Read the model definition and answer for the solid it produces. Units are mm, in the model's axes. Face numbers are marked on the shaded views. A direction names the side the tool comes from. Coordinates: 2 decimals unless noted, no trailing zeros. Write each loop counter-clockwise with the first axis right and the second up, starting at its lowest first coordinate (ties: lowest second). Pieces come first, ordered by that corner, then holes. Notation, with made-up numbers: (-6.5, 83.5) - (36.5, 83.5) arc R19 ccw to (36.5, 100.5) - close; hole circle Ø1 at (1.5, -39). An arc over 180 degrees is marked (long way). Return JSON: item names as keys, results as strings.
```python
from build123d import *

# Parameters (mm, degrees)
SKETCH1_R           = 50
BOSS_EXTRUDE1_DEPTH = 10
SKETCH2_R           = 20
CUT_EXTRUDE1_DEPTH  = 5
CUT_EXTRUDE6_DEPTH  = 3
SKETCH8_R           = 1.7
CUT_EXTRUDE7_DEPTH  = 10
BOSS_EXTRUDE3_DEPTH = 10
CUT_EXTRUDE11_DEPTH = 10
SKETCH15_W          = 131.735170003
SKETCH15_H          = 179.266555965
CUT_EXTRUDE12_DEPTH = 79
BOSS_EXTRUDE4_DEPTH = 4.9
SKETCH17_R          = 1.7
CUT_EXTRUDE13_DEPTH = 10
CUT_EXTRUDE14_DEPTH = 3
SKETCH19_W          = 78.571428572
SKETCH19_H          = 5.1
CUT_EXTRUDE15_DEPTH = 0.5
CUT_EXTRUDE16_DEPTH = 10
CUT_EXTRUDE17_DEPTH = 5.1
SKETCH24_R          = 1.7
CUT_EXTRUDE19_DEPTH = 5.1
SKETCH25_R          = 11
CUT_EXTRUDE20_DEPTH = 7.2
SKETCH26_R          = 9
CUT_EXTRUDE21_DEPTH = 7.2
SKETCH27_R          = 3
CUT_EXTRUDE22_DEPTH = 11
SKETCH28_R          = 1.6
CUT_EXTRUDE23_DEPTH = 12
SKETCH29_R          = 2.9
SKETCH29_R_2        = 1.6
CUT_EXTRUDE24_DEPTH = 3.5
SKETCH30_R          = 12
CUT_EXTRUDE25_DEPTH = 2.4
SKETCH31_R          = 2.8
CUT_EXTRUDE26_DEPTH = 3
FILLET1_R           = 20


with BuildPart() as part:
    # Sketch1 → Boss-Extrude1 (new body)
    with BuildSketch(Plane(origin=(0, 0, 0), x_dir=(1, 0, 0), z_dir=(0, 1, 0))):
        Circle(SKETCH1_R)
    extrude(amount=BOSS_EXTRUDE1_DEPTH)

    # Sketch2 → Cut-Extrude1 (cut)
    with BuildSketch(Plane(origin=(0, 10, 0), x_dir=(1, 0, 0), z_dir=(0, 1, 0))):
        Circle(SKETCH2_R)
    extrude(amount=-CUT_EXTRUDE1_DEPTH, mode=Mode.SUBTRACT)

    # Sketch7 → Cut-Extrude6 (cut)
    with BuildSketch(Plane.XZ):
        with BuildLine():
            ThreePointArc((-2.85, 14.726761355), (0, 15), (2.85, 14.726761355))
            Line((2.85, 14.726761355), (2.85, 16.645448267))
            Line((2.85, 16.645448267), (0, 18.290896534))
            Line((0, 18.290896534), (-2.85, 16.645448267))
            Line((-2.85, 16.645448267), (-2.85, 14.726761355))
        make_face()
        with BuildLine():
            Line((2.85, 13.354551733), (2.85, 14.726761355))
            ThreePointArc((2.85, 14.726761355), (0, 15), (-2.85, 14.726761355))
            Line((-2.85, 14.726761355), (-2.85, 13.354551733))
            Line((-2.85, 13.354551733), (0, 11.709103466))
            Line((0, 11.709103466), (2.85, 13.354551733))
        make_face()
        Polygon((-12.990381057, -4.209103466), (-15.840381057, -5.854551733), (-15.840381057, -9.145448267), (-12.990381057, -10.790896534), (-10.140381057, -9.145448267), (-10.140381057, -5.854551733), align=None)
        Polygon((15.840381057, -5.854551733), (12.990381057, -4.209103466), (10.140381057, -5.854551733), (10.140381057, -9.145448267), (12.990381057, -10.790896534), (15.840381057, -9.145448267), align=None)
    extrude(amount=-CUT_EXTRUDE6_DEPTH, mode=Mode.SUBTRACT)

    # Sketch8 → Cut-Extrude7 (cut)
    with BuildSketch(Plane.XZ):
        with Locations((0, 15)):
            Circle(SKETCH8_R)
        with Locations((12.990381057, -7.5)):
            Circle(SKETCH8_R)
        with Locations((-12.990381057, -7.5)):
            Circle(SKETCH8_R)
    extrude(amount=-CUT_EXTRUDE7_DEPTH, mode=Mode.SUBTRACT)


with BuildPart() as body_2:
    # Sketch9 → Boss-Extrude3 (new body)
    with BuildSketch(Plane.XZ):
        with BuildLine():
            Line((-50, 350), (-50, 0))
            ThreePointArc((-50, 0), (0, 50), (50, 0))
            Line((50, 0), (50, 350))
            Line((50, 350), (-50, 350))
        make_face()
    extrude(amount=-BOSS_EXTRUDE3_DEPTH)

    # Sketch13 → Cut-Extrude11 (cut)
    with BuildSketch(Plane.XZ):
        with BuildLine():
            Line((-50, 350), (-50, 0))
            ThreePointArc((-50, 0), (-49.817332452, 4.270057067), (-49.270664506, 8.5089141))
            Line((-49.270664506, 8.5089141), (-20, 350))
            Line((-20, 350), (-50, 350))
        make_face()
        with BuildLine():
            Line((20, 350), (49.270664506, 8.5089141))
            ThreePointArc((49.270664506, 8.5089141), (49.817332452, 4.270057067), (50, 0))
            Line((50, 0), (50, 350))
            Line((50, 350), (20, 350))
        make_face()
    extrude(amount=-CUT_EXTRUDE11_DEPTH, mode=Mode.SUBTRACT)


with BuildPart() as cut_extrude12_tool:
    # Sketch15 → Cut-Extrude12 (new body)
    with BuildSketch(Plane(origin=(0, 10, 0), x_dir=(1, 0, 0), z_dir=(0, 1, 0))):
        with Locations((-8.166136658, -35.366722018)):
            Rectangle(SKETCH15_W, SKETCH15_H)
    extrude(amount=-CUT_EXTRUDE12_DEPTH)


with BuildPart() as part_1:
    add(part.part)

    # Cut-Extrude12: cut by cut_extrude12_tool
    add(cut_extrude12_tool.part, mode=Mode.SUBTRACT)


with BuildPart() as body_2_1:
    add(body_2.part)

    # Cut-Extrude12: cut by cut_extrude12_tool
    add(cut_extrude12_tool.part, mode=Mode.SUBTRACT)

    # Sketch16 → Boss-Extrude4 (add)
    with BuildSketch(Plane(origin=(0, 10, 0), x_dir=(1, 0, 0), z_dir=(0, 1, 0))):
        Polygon((40.972386827, -105.322153681), (-40.972386827, -105.322153681), (-39.285714286, -125), (39.285714286, -125), align=None)
    extrude(amount=-BOSS_EXTRUDE4_DEPTH)

    # Sketch17 → Cut-Extrude13 (cut)
    with BuildSketch(Plane.XZ.offset(-5.1)):
        with Locations((-25, 115)):
            Circle(SKETCH17_R)
        with Locations((25, 115)):
            Circle(SKETCH17_R)
    extrude(amount=-CUT_EXTRUDE13_DEPTH, mode=Mode.SUBTRACT)

    # Sketch18 → Cut-Extrude14 (cut)
    with BuildSketch(Plane(origin=(0, 10, 0), x_dir=(1, 0, 0), z_dir=(0, 1, 0))):
        Polygon((-25, -111.651368439), (-27.9, -113.325684219), (-27.9, -116.674315781), (-25, -118.348631561), (-22.1, -116.674315781), (-22.1, -113.325684219), align=None)
        Polygon((22.1, -113.325684219), (25, -111.651368439), (27.9, -113.325684219), (27.9, -116.674315781), (25, -118.348631561), (22.1, -116.674315781), align=None)
    extrude(amount=-CUT_EXTRUDE14_DEPTH, mode=Mode.SUBTRACT)

    # Sketch19 → Cut-Extrude15 (cut)
    with BuildSketch(Plane(origin=(0, 0, 125), x_dir=(-1, 0, 0), z_dir=(0, 0, -1))):
        with Locations((0, 2.55)):
            Rectangle(SKETCH19_W, SKETCH19_H)
    extrude(amount=-CUT_EXTRUDE15_DEPTH, mode=Mode.SUBTRACT)

    # Sketch21 → Cut-Extrude16 (cut)
    with BuildSketch(Plane.XZ):
        Polygon((30.285714286, 230), (-30.285714286, 230), (-39.242857143, 125.5), (39.242857143, 125.5), align=None)
        Polygon((-30.285714286, 230), (-45.620097138, 230), (-45.620097138, 89.112609713), (46.495880164, 89.112609713), (46.495880164, 230), (30.285714286, 230), (39.242857143, 125.5), (-39.242857143, 125.5), align=None)
    extrude(amount=-CUT_EXTRUDE16_DEPTH, mode=Mode.SUBTRACT)

    # Sketch21_3 → Cut-Extrude17 (cut)
    with BuildSketch(Plane.XZ):
        Polygon((-28.571428571, 250), (-30.285714286, 230), (30.285714286, 230), (28.571428571, 250), align=None)
    extrude(amount=-CUT_EXTRUDE17_DEPTH, mode=Mode.SUBTRACT)

    # Sketch24 → Cut-Extrude19 (cut)
    with BuildSketch(Plane.XZ.offset(-5.1)):
        with Locations((20, 240)):
            Circle(SKETCH24_R)
        with Locations((-20, 240)):
            Circle(SKETCH24_R)
    extrude(amount=-CUT_EXTRUDE19_DEPTH, mode=Mode.SUBTRACT)

    # Sketch25 → Cut-Extrude20 (cut)
    with BuildSketch(Plane.XZ):
        with Locations((0, 330)):
            Circle(SKETCH25_R)
    extrude(amount=-CUT_EXTRUDE20_DEPTH, mode=Mode.SUBTRACT)

    # Sketch26 → Cut-Extrude21 (cut)
    with BuildSketch(Plane.XZ.offset(-7.2)):
        with Locations((0, 330)):
            Circle(SKETCH26_R)
    extrude(amount=-CUT_EXTRUDE21_DEPTH, mode=Mode.SUBTRACT)

    # Sketch27 → Cut-Extrude22 (cut)
    with BuildSketch(Plane.XZ):
        with Locations((0, 270)):
            Circle(SKETCH27_R)
    extrude(amount=-CUT_EXTRUDE22_DEPTH, mode=Mode.SUBTRACT)

    # Sketch28 → Cut-Extrude23 (cut)
    with BuildSketch(Plane(origin=(0, 10, 0), x_dir=(1, 0, 0), z_dir=(0, 1, 0))):
        with Locations((-15.5, -254.5)):
            Circle(SKETCH28_R)
        with Locations((15.5, -254.5)):
            Circle(SKETCH28_R)
        with Locations((15.5, -285.5)):
            Circle(SKETCH28_R)
        with Locations((-15.5, -285.5)):
            Circle(SKETCH28_R)
    extrude(amount=-CUT_EXTRUDE23_DEPTH, mode=Mode.SUBTRACT)

    # Sketch29 → Cut-Extrude24 (cut)
    with BuildSketch(Plane.XZ):
        with Locations((-15.5, 285.5)):
            Circle(SKETCH29_R)
        with Locations((-15.5, 285.5)):
            Circle(SKETCH29_R_2, mode=Mode.SUBTRACT)
        with Locations((15.5, 285.5)):
            Circle(SKETCH29_R)
        with Locations((15.5, 254.5)):
            Circle(SKETCH29_R)
        with Locations((-15.5, 254.5)):
            Circle(SKETCH29_R)
    extrude(amount=-CUT_EXTRUDE24_DEPTH, mode=Mode.SUBTRACT)

    # Sketch30 → Cut-Extrude25 (cut)
    with BuildSketch(Plane(origin=(0, 10, 0), x_dir=(1, 0, 0), z_dir=(0, 1, 0))):
        with Locations((0, -270)):
            Circle(SKETCH30_R)
    extrude(amount=-CUT_EXTRUDE25_DEPTH, mode=Mode.SUBTRACT)

    # Sketch31 → Cut-Extrude26 (cut)
    with BuildSketch(Plane(origin=(0, 10, 0), x_dir=(1, 0, 0), z_dir=(0, 1, 0))):
        with Locations((-20, -240)):
            Circle(SKETCH31_R)
        with Locations((20, -240)):
            Circle(SKETCH31_R)
    extrude(amount=-CUT_EXTRUDE26_DEPTH, mode=Mode.SUBTRACT)

    # Fillet1
    fillet1_edges = [body_2_1.edges().sort_by_distance(p)[0] for p in [
        (-20, 5, 350),
        (20, 5, 350),
    ]]
    fillet(fillet1_edges, radius=FILLET1_R)


solid = body_2_1.part
```
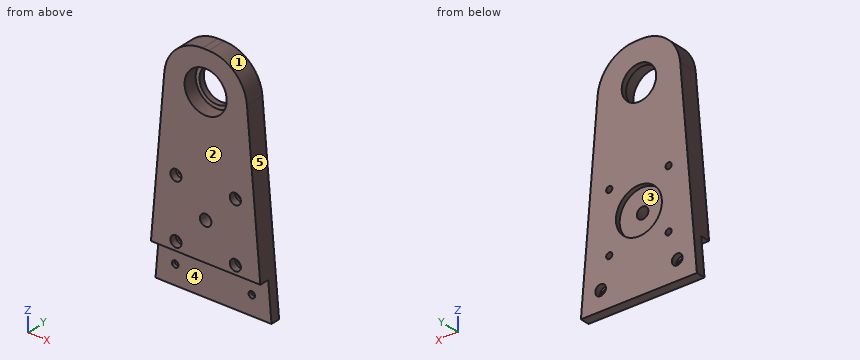
(1) A cutting plane is placed at C-C (z = 270). Determine the outline of the cut face in (x, y).
Answer:
{"outline": "(-26.86, 0) - (-3, 0) - (-3, 7.6) - (-12, 7.6) - (-12, 10) - (-26.86, 10) - close; (3, 0) - (26.86, 0) - (26.86, 10) - (12, 10) - (12, 7.6) - (3, 7.6) - close"}
(2) A cutting plane is placed at D-D (x = 15.5). Determine the outline of the cut face in (y, z).
Answer:
{"outline": "(0, 250) - (5.1, 250) - (5.1, 230) - (10, 230) - (10, 252.9) - (3.5, 252.9) - (3.5, 251.6) - (0, 251.6) - close; (0, 257.4) - (3.5, 257.4) - (3.5, 256.1) - (10, 256.1) - (10, 283.9) - (3.5, 283.9) - (3.5, 282.6) - (0, 282.6) - close; (0, 288.4) - (3.5, 288.4) - (3.5, 287.1) - (10, 287.1) - (10, 344.42) - (0, 344.42) - close"}
(3) A cutting plane is placed at B-B (z = 240). Determine the outline of the cut face in (x, y), and give its area (3 significant figures).
Answer:
{"outline": "(-29.43, 5.1) - (-21.7, 5.1) - (-21.7, 7) - (-22.8, 7) - (-22.8, 10) - (-29.43, 10) - close; (-18.3, 5.1) - (18.3, 5.1) - (18.3, 7) - (17.2, 7) - (17.2, 10) - (-17.2, 10) - (-17.2, 7) - (-18.3, 7) - close; (21.7, 5.1) - (29.43, 5.1) - (29.43, 10) - (22.8, 10) - (22.8, 7) - (21.7, 7) - close", "area": "242 mm²"}
(4) Determine the mould class of the marked faces 1, 2 and 3 for opening direction X: +X half, -X half, draft (parallel to the pull), parting line (faces both ways), or undercut.
Answer:
{"face 1": "+X half", "face 2": "draft", "face 3": "undercut"}
(5) Flat-ended cylindrical pins translate along their axes: P1, Ø12, axis at x = 15.5, z = 262.5, coming from the -Y side; P2, Ø3, axis at x = 19, z = 239.5, coming from the +Y side; P3, Ø3, axis at x = 15, z = 255, coming from the -Y side; P4, Ø3, axis at y = 2.5, z = 285, coming from the +X side. Find the tip coordinate at first contact, or state that the pin passes through.
Answer:
{"P1": "y = 0", "P2": "y = 7", "P3": "y = 3.5", "P4": "x = 25.7"}
(6) Straight lines are drawn through the part: line 1 (Z direction, x = 0, y = 5.5); line 2 (Z direction, x = 0, y = 2.5); line 3 (X direction, y = 6.1, z = 240). For each, find the intervals that lie inside material, in ascending order. Write a range as from..to.
Answer:
{"line 1": "230..267, 273..319, 341..350", "line 2": "250..267, 273..319, 341..350", "line 3": "-29.43..-21.7, -18.3..18.3, 21.7..29.43"}
(7) A cutting plane is placed at A-A (x = 0). Determine the outline of the cut face in (y, z).
Answer:
{"outline": "(0, 250) - (5.1, 250) - (5.1, 230) - (10, 230) - (10, 258) - (7.6, 258) - (7.6, 267) - (0, 267) - close; (0, 273) - (7.6, 273) - (7.6, 282) - (10, 282) - (10, 321) - (7.2, 321) - (7.2, 319) - (0, 319) - close; (0, 341) - (7.2, 341) - (7.2, 339) - (10, 339) - (10, 350) - (0, 350) - close"}
(8) Which of the six approach directions +Z, -Z, +X, -X, +Y, -Y give full straight-line access (tool end or side, diameter ignored) to the marked faces 4 and 5?
Answer:
{"face 4": "-Z, +X, -X, -Y", "face 5": "+Z, +X, +Y, -Y"}
